Model file for the job. Use its own axes, mm. Face numbers are marked on the shaded views. A direction names the side the tool comes from. Coordinates: 2 decimals unless noted, no trailing zeros. Order: outer loops, then holes, each group sorted by start corner. A loop starts at its lowest first (then second) coordinate and runs counter-clockwise, first axis right, second up. Notation, with made-up numbers: (-12.5, 75) -> (22.5, 75) arc R23 ccw to (22.5, 105) -> close; hole circle Ø11 at (59, 21.5). An arc over 180 degrees is marked (long way). Write item = value, one per line. Start each with the question number.
Q1. Flat gauge pins, fed straight in: pin 1 (10 mm diameter, centred on x = 8, z = -0.5, fed in from +Y); pin 2 (4 mm diameter, centred on y = 17.5, z = -11, fed in from +X); pin 3 (1.5 mm diameter, centred on x = 0.5, z = 2, fed in from +Y); pin 4 (12 mm diameter, centred on x = -7, y = 32, fed in from +Z). Where does each tip first touch, or does it go through?
Q2. 3-axis set-ups, long thin cutter, end or side, ignore diameter. For the marked faces 1 and 2: which of +Z, -Z, +X, -X, +Y, -Y reach the whole face in a straight line?
Q3. Cut at A-A, the plane y = 16. List the corners of the cut face in (x, z), plus the area to 3 significant figures.
Q4. Cut at B-B, the plane y = 26. List the corners of the cut face in (x, z).
Q5. Wall check: line 1 (Z direction, x = -2, y = 27.5); line 2 (Z direction, x = -5, y = 33.5); line 3 (X direction, y = 39.5, z = -5). Give the ranges that are in metal, low to high. Write a range as from..to.
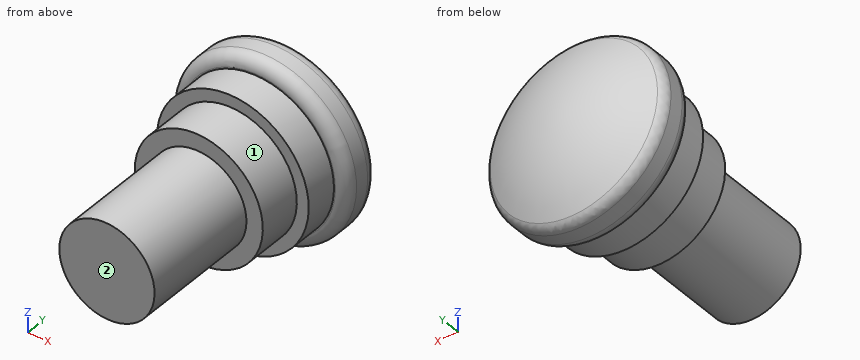
from build123d import *

# Parameters (mm, degrees)
FILLET1_R = 2


with BuildPart() as part:
    # Sketch1 → Revolve1 (revolve)
    with BuildSketch(Plane(origin=(0, 0, 0), x_dir=(0, 0, -1), z_dir=(1, 0, 0))):
        with BuildLine():
            Line((15, 38.4), (15, 32.9))
            Line((15, 32.9), (12.75, 32.9))
            Line((12.75, 32.9), (12.75, 27.4))
            Line((12.75, 27.4), (10.75, 27.4))
            Line((10.75, 27.4), (10.75, 20))
            Line((10.75, 20), (8, 20))
            Line((8, 20), (8, 0))
            Line((8, 0), (0, 0))
            Line((0, 0), (0, 43))
            ThreePointArc((0, 43), (7.844743463, 41.824163466), (15, 38.4))
        make_face()
    revolve(axis=Axis((0, 43, 0), (0, -1, 0)))

    # Fillet1
    fillet1_edges = [part.edges().sort_by_distance(p)[0] for p in [
        (0, 32.9, 15),
        (0, 38.4, 15),
    ]]
    fillet(fillet1_edges, radius=FILLET1_R)


solid = part.part
Here are the results:
q1.pin_1 = 42.83
q1.pin_2 = through
q1.pin_3 = 42.97
q1.pin_4 = 14.9
q2.face_1 = -Y
q2.face_2 = +Z, -Z, +X, -X, -Y
q3.outline = circle Ø16 at (0, 0)
q3.area = 201 mm²
q4.outline = circle Ø21.5 at (0, 0)
q5.line_1 = -12.59..12.59
q5.line_2 = -13.53..13.53
q5.line_3 = -12.25..12.25
